The figure shows three views and two pictorial views of one solid part (mm, origin at its lowest corner). Answer the questions. Coordinates: 2 decimals unless noted, no trailing zeros. Loops run counter-clockwise (first coordinate to the right, second up) from the corner with the lowest first, then second, coordinate; pieces in that order, holes last. Notation, with made-up numbers: M 47,53 L 99,53 A21 ccw 99,92 Z; hole C 27,-8.5 d10. An arc over 180 degrees is marked long. Answer in a Markdown table with one row per item. Add a question column.
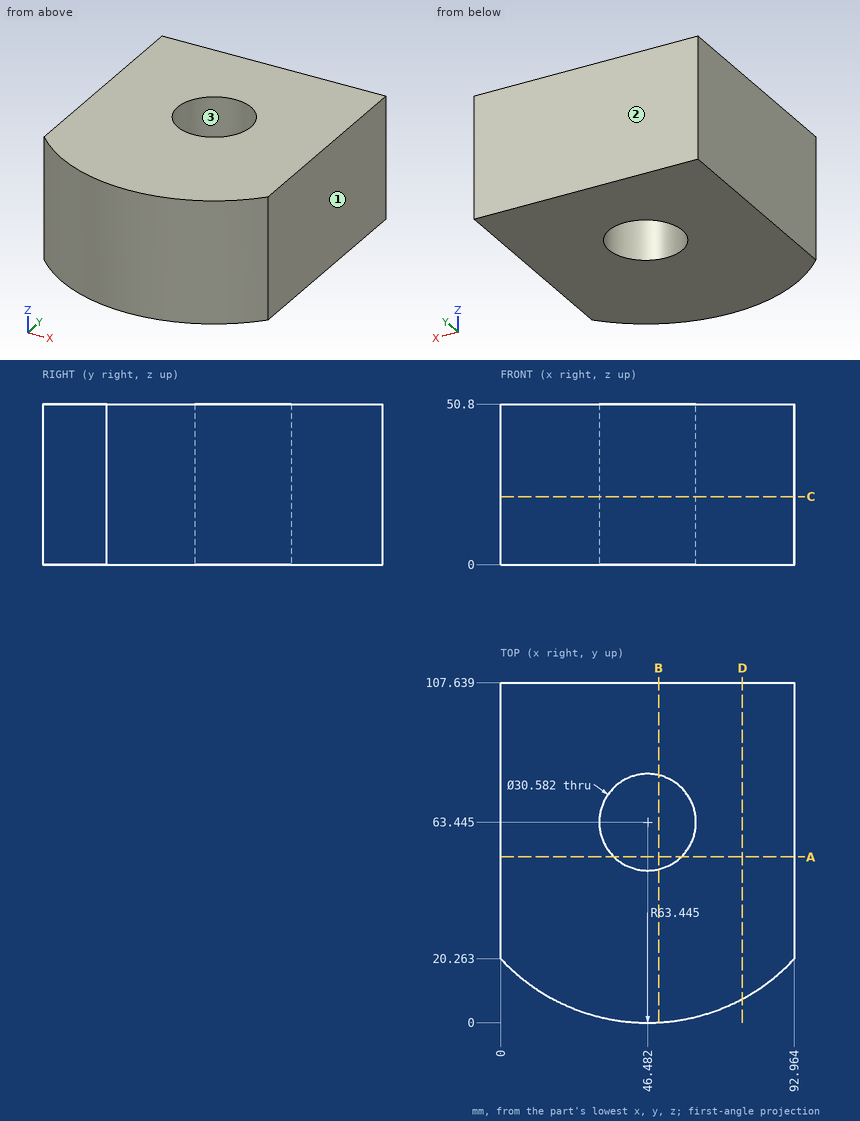
(1) A cutting plane is placed at A-A (y = 52.5). Give the vertices of the cut face in (x, z).
(2) Each of these flat-tipped pins is pushed along its axis until it touches: pin 1 (6 mm diameter, centred on x = 73.5, z = 33.5, fed in from -Y); pin 2 (6 mm diameter, centred on x = 57.5, z = 40.5, fed in from -Y); pin 3 (1 mm diameter, centred on x = 11, z = 38, fed in from -Y) (1 decimal). Where does it stop, or does it pass through?
(3) A cutting plane is placed at D-D (x = 76.5). Give the vertices of the cut face in (y, z), plus the area to 3 significant figures.
(4) A cutting plane is placed at C-C (z = 21.5). Give the vertices of the cut face in (x, y) (1 decimal), plus the area to 3 significant figures.
(5) Straight lines are drawn through the part: line 1 (Y direction, x = 54, z = 8); line 2 (X direction, y = 71, z = 34) (1 decimal); line 3 (Y direction, x = 38.5, z = 36) (1 decimal). For each, find the intervals that lie inside material, in ascending order.
(6) The mould has two halves that part along Y. Classify the marked faces 1, 2 and 3: released by +Y, released by -Y, zero draft, split by the parting line, or undercut.
(7) A cutting plane is placed at B-B (x = 50). Give the vertices of the cut face in (y, z) (1 decimal).
Solved:
| question | item | result |
|---|---|---|
| 1 | outline | M 0,0 L 35.8,0 L 35.8,50.8 L 0,50.8 Z; M 57.16,0 L 92.96,0 L 92.96,50.8 L 57.16,50.8 Z |
| 2 | pin 1 | stops at y = 4.72 |
| 2 | pin 2 | stops at y = 0.51 |
| 2 | pin 3 | stops at y = 10.5 |
| 3 | outline | M 7.55,0 L 107.64,0 L 107.64,50.8 L 7.55,50.8 Z |
| 3 | area | 5,080 mm² |
| 4 | outline | M 0,20.3 A63.4 ccw 93,20.3 L 93,107.6 L 0,107.6 Z; hole C 46.5,63.4 d30.6 |
| 4 | area | 8,690 mm² |
| 5 | line 1 | y = 0.45 to 50.13, 76.76 to 107.64 |
| 5 | line 2 | x = 0 to 33.2, 59.8 to 93 |
| 5 | line 3 | y = 0.5 to 50.4, 76.5 to 107.6 |
| 6 | face 1 | zero draft |
| 6 | face 2 | released by +Y |
| 6 | face 3 | undercut |
| 7 | outline | M 0.1,0 L 48.6,0 L 48.6,50.8 L 0.1,50.8 Z; M 78.3,0 L 107.6,0 L 107.6,50.8 L 78.3,50.8 Z |
